Autodesk Inventor part; units mm, degrees
ref_plane "YZ Plane" through (0, 0, 0) normal (1, 0, 0) x (0, 1, 0)
ref_plane "XZ Plane" through (0, 0, 0) normal (0, 1, 0) x (-1, 0, 0)
ref_plane "XY Plane" through (0, 0, 0) normal (0, 0, 1) x (1, 0, 0)
sketch "Эскиз1" plane through (0, 0, 0) normal (0, 1, 0) x (-1, 0, 0)
  circle A0 centre (16.875, 37.75) radius 1.6
  circle A1 centre (-30.625, 37.75) radius 1.6
  line L0 (-35, 40.5) -> (27, 40.5)
  line L1 (-35, 35) -> (-35, 40.5)
  line L2 (27, 35) -> (-35, 35)
  line L3 (27, 40.5) -> (27, 35)
  circle A2 centre (16.875, -37.75) radius 1.6
  circle A3 centre (-30.625, -37.75) radius 1.6
  line L4 (-35, -40.5) -> (27, -40.5)
  line L5 (27, -40.5) -> (27, -35)
  line L6 (-35, -35) -> (27, -35)
  line L7 (-35, -35) -> (-35, -40.5)
  line L8 (35, -35) -> (27, -35)
  line L9 (35, -35) -> (35, -20)
  line L10 (35, -20) -> (35, 20)
  line L11 (35, 20) -> (35, 35)
  line L12 (35, 35) -> (27, 35)
  line L13 (-35, 20) -> (-35, -20)
  line L14 (-35, 35) -> (-35, 20)
  line L15 (-35, -20) -> (-35, -35)
  point P0 (0, 0)
  point P1 (0, 0)
extrude "Выдавливание1" add sketch "Эскиз1" along normal blind 3
sketch "Эскиз2" plane through (0, 3, 0) normal (0, 1, 0) x (1, 0, 0)
  line L0 (-21.5, -21.875) -> (-21.5, 21.875)
  line L1 (21.5, -21.875) -> (-21.5, -21.875)
  line L2 (21.5, 21.875) -> (21.5, -21.875)
  line L3 (-21.5, 21.875) -> (21.5, 21.875)
  circle A0 centre (18.5, -18.5) radius 1.5
  circle A1 centre (-18.5, -18.5) radius 1.5
  circle A2 centre (-18.5, 18.5) radius 1.5
  circle A3 centre (18.5, 18.5) radius 1.5
  point P0 (0, 0)
  point P1 (0, 0)
extrude "Выдавливание2" cut sketch "Эскиз2" against normal blind 10 contours A0 | A1 | A2 | A3
properties part number "000,105 - Дно переднего сегмента"
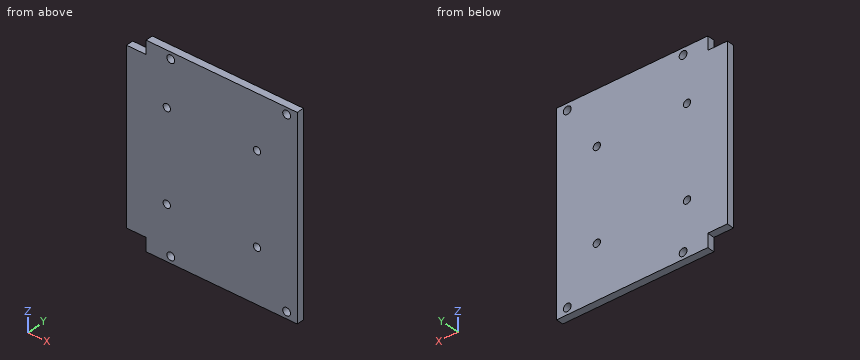
Model file for the job. Use its own axes, mm. Coordinates: 2 decimals unless noted, no trailing zeros. Loops run counter-clockwise (first coordinate to the right, second up) from the corner with the lowest first, then second, coordinate; pieces in that order, holes last. Notation, with made-up numbers: (6.25, 9) - (65.25, 9) arc R17 ccw to (65.25, 21) - close; hole circle Ø4 at (47, -33.75). An arc over 180 degrees is marked (long way). Answer as a JSON object with one key per item and string values. Group by question number.
(1) Flat gauge pins, fed straight in: pin 1 (4 mm diameter, centred on x = 18.5, z = -18.5, fed in from +Y); pin 2 (0.9 mm diameter, centred on y = 1, z = 38.5, fed in from -X); pin 3 (1.5 mm diameter, centred on x = -30, y = 2, fed in from +Z). Where does each tip first touch, or does it go through?
(2) Cut at B-B (x = 18.5). Give the cut face in (y, z), then the cut area to 3 significant figures.
(3) Cut at C-C (y = 1.85). State how many separate pieces and enclosed holes the cut face has, then the cut area to 3 significant figures.
(4) Probe line 1 along Z through (x, y) = (18.5, 2.1); line 2 along Z through (x, y) = (-15.5, 2.4); line 3 along X through (y, z) = (1.35, -19.5). List the from-to ranges inside material, lowest first.
(5) Cut at A-A (z = -37.75). Give the cut face in (x, y) (3 decimals).
Geometry says:
{
 "1": {"pin 1": "stops at y = 3", "pin 2": "stops at x = -27", "pin 3": "stops at z = 35"},
 "2": {"outline": "(0, -40.5) - (3, -40.5) - (3, -20) - (0, -20) - close; (0, -17) - (3, -17) - (3, 17) - (0, 17) - close; (0, 20) - (3, 20) - (3, 40.5) - (0, 40.5) - close", "area": "225 mm^2"},
 "3": {"separate pieces": "1", "enclosed holes": "8", "area": "5,520 mm^2"},
 "4": {"line 1": "z = -40.5 to -20, -17 to 17, 20 to 40.5", "line 2": "z = -40.5 to -38.57, -36.93 to 36.93, 38.57 to 40.5", "line 3": "x = -35 to -19.62, -17.38 to 17.38, 19.62 to 35"},
 "5": {"outline": "(-27, 0) - (-18.475, 0) - (-18.475, 3) - (-27, 3) - close; (-15.275, 0) - (29.025, 0) - (29.025, 3) - (-15.275, 3) - close; (32.225, 0) - (35, 0) - (35, 3) - (32.225, 3) - close"}
}
